from build123d import *

# Parameters (mm, degrees)
SKETCH026_R     = 3.8
PAD009_DEPTH    = 3
SKETCH027_R     = 3.2
PAD010_DEPTH    = 2.6
FILLET_R        = 1
SKETCH029_R     = 2
POCKET013_DEPTH = 1


with BuildPart() as part:
    # Sketch026 → Pad009 (new body)
    with BuildSketch(Plane.XZ):
        with Locations((28.8, 9.2)):
            Circle(SKETCH026_R)
    extrude(amount=PAD009_DEPTH)

    # Sketch027 (on Face3 of Pad009) → Pad010 (join)
    with BuildSketch(Plane.XZ.offset(3)):
        with Locations((28.8, 9.2)):
            Circle(SKETCH027_R)
    extrude(amount=PAD010_DEPTH)

    # Fillet
    fillet_edges = [part.edges().sort_by_distance(p)[0] for p in [
        (25.6, -5.6, 9.2),
    ]]
    fillet(fillet_edges, radius=FILLET_R)

    # Sketch029 (on Face6 of Fillet) → Pocket013 (cut)
    with BuildSketch(Plane(origin=(0, 0, 0), x_dir=(1, 0, 0), z_dir=(0, 1, 0))):
        with Locations((28.8, -9.2)):
            Circle(SKETCH029_R)
    extrude(amount=-POCKET013_DEPTH, mode=Mode.SUBTRACT)


with BuildPart() as part_1:
    # Body003 placement: moved
    add(part.part.moved(Location((0, 1.4, 0))))


solid = part_1.part
Part model, mm, in its own coordinate system. A direction names the side the tool comes from. Give positions to 0.01 mm unless a question says otherwise; leave off trailing zeros. Order: outer loops, then holes, each group sorted by start corner. A loop starts at its lowest first (then second) coordinate and runs counter-clockwise, first axis right, second up. Notation, with made-up numbers: (45, -37) -> (81, -37) arc R22 ccw to (81, 0) -> close; hole circle Ø6 at (-6.5, -9.75). An arc over 180 degrees is marked (long way). Use one line per item in the form item = value.
(1) Drill centre lines: line 1 (Z direction, x = 28.8, y = 1.1); line 2 (Y direction, x = 28, z = 9.5); line 3 (X direction, y = 0.55, z = 11.25). Where is each one in solid material? Low to high. Write a range as from..to.
Solution:
line_1 = 5.4..7.2, 11.2..13
line_2 = -4.2..0.4
line_3 = 25.6..32
(2) Pull direction X, two halves, no side cores. Call faces 1 (the face through (29, -4.2, 9)), 2 (the face through (29, 0.4, 9)), 3 (the face through (31.852, -2.389, 10.161)): +X half, -X half, draft (parallel to the pull), parting line (faces both ways), or undercut.
Solution:
face_1 = draft
face_2 = undercut
face_3 = parting line
(3) Tool access for faces 4 (the face through (25.004, -0.079, 9.367)), 5 (the face through (30, -1.6, 6)), 6 (the face through (27.2, 0.9, 10.4)): list every direction of +Z, -Z, +X, -X, +Y, -Y with a clear straight run to the whole face (end or side of a thin tool).
Solution:
face_4 = +Y, -Y
face_5 = -Y
face_6 = +Y
(4) Saw through at A-A (x = 28.8). Write the cut outline in (y, z), then the cut area to 3 significant figures.
Solution:
outline = (-4.2, 7) arc R1 ccw to (-3.2, 6) -> (-1.6, 6) -> (-1.6, 5.4) -> (1.4, 5.4) -> (1.4, 7.2) -> (0.4, 7.2) -> (0.4, 11.2) -> (1.4, 11.2) -> (1.4, 13) -> (-1.6, 13) -> (-1.6, 12.4) -> (-3.2, 12.4) arc R1 ccw to (-4.2, 11.4) -> close
area = 35.0 mm²
(5) Saw through at C-C (y = -0.7). Write the cut outline in (x, z).
Solution:
outline = circle Ø7.6 at (28.8, 9.2)
(6) Flat gauge pins, fed straight in: P1, Ø1.5, axis at x = 27.5, y = -2.5, coming from the -Z side; P2, Ø1.2, axis at x = 28, z = 9, coming from the +Y side. Where does each tip first touch, or does it go through?
Solution:
P1 = 6.05
P2 = 0.4
(7) Saw through at B-B (z = 9.2). Write the cut outline in (x, y).
Solution:
outline = (25, -1.6) -> (25.6, -1.6) -> (25.6, -3.2) arc R1 ccw to (26.6, -4.2) -> (31, -4.2) arc R1 ccw to (32, -3.2) -> (32, -1.6) -> (32.6, -1.6) -> (32.6, 1.4) -> (30.8, 1.4) -> (30.8, 0.4) -> (26.8, 0.4) -> (26.8, 1.4) -> (25, 1.4) -> close
